The model under review builds one solid part; all positions refer to its coordinate system, in mm. Face numbers are marked on the shaded views. Round coordinates to 2 decimals unless told otherwise and drop trailing zeros. Write each loop counter-clockwise with the first axis right and the second up, starting at its lowest first coordinate (ties: lowest second). Pieces come first, ordered by that corner, then holes. Notation, with made-up numbers: (-33.75, -9.75) -> (-15.75, -9.75) arc R20 cw to (-15.75, -0.75) -> close; hole circle Ø8 at (21.5, -32). An arc over 180 degrees is marked (long way). Answer as a JSON object with one key per item and string values. Group by question number.
1) To check wall thickness, follow probe 1 along Z at (x, y) = (-25, 14); probe 2 along Y at (x, z) = (-24, 20); probe 3 along X at (y, z) = (5.5, 11.5). State the ranges of each line that lie inside material, in increasing order. Write a range as [from, to].
2) We need section A-A, the plane z = 11. Write out the cut boundary in (x, y), then the cut area to 3 significant figures.
3) Mouldability with a two-part tool opening along Z and no side actions: class the marked faces 1, 2, 3 and 4 as pulls with the +Z half, pulls with the -Z half, needs draft (parallel to the pull), parting line crosses it, or undercut.
4) We need section B-B, the plane x = 25. Write out the cut boundary in (y, z).
5) We need section C-C, the plane y = -18.5. Write out the cut boundary in (x, z), then the cut area to 3 significant figures.
6) We need section D-D, the plane x = 0. Write out the cut boundary in (y, z).
7) Insertion check: pin 1 Ø12 at (x, y) = (2.5, 12) entering from -Z. The pin has a flat end and moves straight along its axis. Give the tip position at first contact, or say it passes through.
from build123d import *

# Parameters (mm, degrees)
F0_W     = 60
F0_H     = 60
F0_R     = 20
F1_DEPTH = 60
F2_W     = 10.025016
F2_H     = 2
F3_DEPTH = 60.001
F4_R     = 4
F5_DEPTH = 60


with BuildPart() as f1:
    # F0 (on Top) → F1 (new body)
    with BuildSketch(Plane.XY):
        Rectangle(F0_W, F0_H)
        Circle(F0_R, mode=Mode.SUBTRACT)
    extrude(amount=F1_DEPTH)

    # F2 (on face) → F3 (cut, through all)
    with BuildSketch(Plane.XY.offset(60)):
        with Locations((-24.987492, 0)):
            Rectangle(F2_W, F2_H)
    extrude(amount=-F3_DEPTH, mode=Mode.SUBTRACT)

    # F4 (on face) → F5 (cut)
    with BuildSketch(Plane(origin=(0, 30, 0), x_dir=(-1, 0, 0), z_dir=(0, 1, 0))):
        with Locations((25, 11)):
            Circle(F4_R)
        with Locations((25, 49)):
            Circle(F4_R)
        with Locations((-25, 49)):
            Circle(F4_R)
        with Locations((-25, 11)):
            Circle(F4_R)
    extrude(amount=-F5_DEPTH, mode=Mode.SUBTRACT)


solid = f1.part
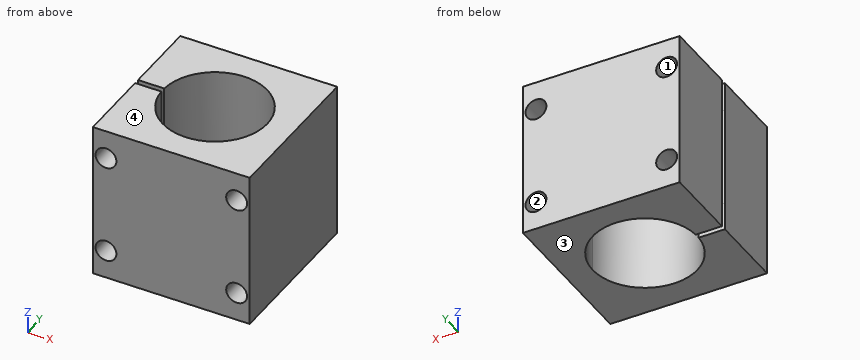
Here are the results:
{
 "1": {"probe 1": "z = [0, 7], [15, 45], [53, 60]", "probe 2": "y = [-30, -1], [1, 30]", "probe 3": "x = [-30, -28.97], [-21.03, -19.23], [19.23, 21.03], [28.97, 30]"},
 "2": {"outline": "(-30, -30) -> (-29, -30) -> (-29, -1) -> (-30, -1) -> close; (-30, 1) -> (-29, 1) -> (-29, 30) -> (-30, 30) -> close; (-21, -30) -> (21, -30) -> (21, 30) -> (-21, 30) -> (-21, 1) -> (-19.97, 1) arc R20 cw (long way) to (-19.97, -1) -> (-21, -1) -> close; (29, -30) -> (30, -30) -> (30, 30) -> (29, 30) -> close", "area": "1,380 mm^2"},
 "3": {"face 1": "undercut", "face 2": "undercut", "face 3": "pulls with the -Z half", "face 4": "pulls with the +Z half"},
 "4": {"outline": "(-30, 0) -> (30, 0) -> (30, 7) -> (-30, 7) -> close; (-30, 15) -> (30, 15) -> (30, 45) -> (-30, 45) -> close; (-30, 53) -> (30, 53) -> (30, 60) -> (-30, 60) -> close"},
 "5": {"outline": "(-30, 0) -> (-7.6, 0) -> (-7.6, 60) -> (-30, 60) -> close; (7.6, 0) -> (30, 0) -> (30, 60) -> (7.6, 60) -> close; hole circle Ø8 at (-25, 11); hole circle Ø8 at (-25, 49); hole circle Ø8 at (25, 11); hole circle Ø8 at (25, 49)", "area": "2,490 mm^2"},
 "6": {"outline": "(-30, 0) -> (-20, 0) -> (-20, 60) -> (-30, 60) -> close; (20, 0) -> (30, 0) -> (30, 60) -> (20, 60) -> close"},
 "7": {"pin 1": "passes through"}
}
